Check sheet for the modelled part. Datum: model origin and axes. Units: mm. Give positions to 0.01 mm unless a question says otherwise; leave off trailing zeros. Order: outer loops, then holes, each group sorted by start corner. A loop starts at its lowest first (then second) coordinate and runs counter-clockwise, first axis right, second up.
Item 1: Material ranges on line 1 along Z through (x, y) = (158, -125); line 2 along Z through (x, y) = (-2.5, -259.5); line 3 along Y through (x, z) = (3, 0), recorded low to high.
Item 2: Sectioned sample at B-B on y = -274. Record the boundary of the cut face in (x, z), and give its area (3 significant figures).
Item 3: Gauge pin test, flat ends, axial feed: P1, Ø0.5, axis at x = 55, z = 0, coming from the -Y side; P2, Ø6, axis at y = -262.5, z = -4.5, coming from the -X side; P3, Ø3, axis at y = -393.5, z = -0.5, coming from the +X side; P4, Ø5, axis at x = 116, z = 5, coming from the +Y side. Record the tip position at first contact, or that the pin passes through.
Item 4: Sectioned sample at A-A on x = 101. Record the boundary of the cut face in (y, z).
Item 5: Sectioned sample at C-C on x = 163. Record the boundary of the cut face in (y, z), and give its area (3 significant figures).
from build123d import *

# Parameters (mm, degrees)
BOSS_EXTRUDE1_DEPTH      = 0.5
BOSS_EXTRUDE1_DEPTH_BACK = 0.5
SKETCH2_R                = 3
BOSS_EXTRUDE2_DEPTH      = 600


with BuildPart() as part:
    # Sketch1 → Boss-Extrude1 (new, two sides: drawn at the far end of the back side and taken through both)
    with BuildSketch(Plane.XY.offset(-BOSS_EXTRUDE1_DEPTH_BACK)):
        Polygon((0, 0), (0, -140), (200, -140), align=None)
    extrude(amount=BOSS_EXTRUDE1_DEPTH + BOSS_EXTRUDE1_DEPTH_BACK)

    # Sketch2 → Boss-Extrude2 (add)
    with BuildSketch(Plane(origin=(0, 0, 0), x_dir=(1, 0, 0), z_dir=(0, 1, 0))):
        with Locations(Location((0, 0.5, 0), (0, 0, 270))):
            Circle(SKETCH2_R)
    extrude(amount=-BOSS_EXTRUDE2_DEPTH)

    # Sketch3 → Revolve1 (revolve)
    with BuildSketch(Plane.XY):
        with BuildLine():
            Line((0, 12), (0, -12))
            ThreePointArc((0, -12), (-12, 0), (0, 12))
        make_face()
    revolve(axis=Axis((0, 12, 0), (0, -1, 0)))


solid = part.part
Report:
1. line 1: z = -0.5 to 0.5
1. line 2: z = -2.16 to 1.16
1. line 3: y = -140 to 11.62
2. outline: circle Ø6 at (0, -0.5)
2. area: 28.3 mm2
3. P1: stops at y = -140
3. P2: stops at x = -2.83
3. P3: stops at x = 3
3. P4: passes through
4. outline: (-140, -0.5) - (-70.7, -0.5) - (-70.7, 0.5) - (-140, 0.5) - close
5. outline: (-140, -0.5) - (-114.1, -0.5) - (-114.1, 0.5) - (-140, 0.5) - close
5. area: 25.9 mm2
